```python
from build123d import *

# Parameters (mm, degrees)
SKETCH1_W           = 25.4
SKETCH1_H           = 88.9
BOSS_EXTRUDE1_DEPTH = 30.226
SKETCH2_R           = 3.175
CUT_EXTRUDE1_DEPTH  = 12.7
SKETCH3_R           = 8.763
CUT_EXTRUDE2_DEPTH  = 3.556
CUT_EXTRUDE3_START  = -21.844
SKETCH4_R           = 10.795
CUT_EXTRUDE3_DEPTH  = 21.844
SKETCH5_W           = 54.61
SKETCH5_H           = 30.226
BOSS_EXTRUDE2_DEPTH = 3.175
SKETCH6_R           = 1.5875
CUT_EXTRUDE4_DEPTH  = 3.175
BOSS_EXTRUDE3_START = 2.54
SKETCH8_R           = 10.795
SKETCH8_R_2         = 6.35
BOSS_EXTRUDE3_DEPTH = 2.54


with BuildPart() as part:
    # Sketch1 → Boss-Extrude1 (new body)
    with BuildSketch(Plane.XY):
        Rectangle(SKETCH1_W, SKETCH1_H)
    extrude(amount=BOSS_EXTRUDE1_DEPTH)

    # Sketch2 → Cut-Extrude1 (cut)
    with BuildSketch(Plane(origin=(12.7, 0, 0), x_dir=(0, 0, -1), z_dir=(1, 0, 0))):
        with Locations((-15.113, 38.1)):
            Circle(SKETCH2_R)
        with Locations((-15.113, -38.1)):
            Circle(SKETCH2_R)
    extrude(amount=-CUT_EXTRUDE1_DEPTH, mode=Mode.SUBTRACT)

    # Sketch3 → Cut-Extrude2 (cut)
    with BuildSketch(Plane(origin=(12.7, 0, 0), x_dir=(0, 0, -1), z_dir=(1, 0, 0))):
        with Locations((-15.113, 0)):
            Circle(SKETCH3_R)
    extrude(amount=-CUT_EXTRUDE2_DEPTH, mode=Mode.SUBTRACT)

    # Sketch4 → Cut-Extrude3 (cut)
    with BuildSketch(Plane(origin=(9.144, 0, 0), x_dir=(0, 0, -1), z_dir=(1, 0, 0)).offset(CUT_EXTRUDE3_START)):
        with Locations((-15.113, 0)):
            Circle(SKETCH4_R)
    extrude(amount=CUT_EXTRUDE3_DEPTH, mode=Mode.SUBTRACT)

    # Sketch5 → Boss-Extrude2 (add)
    with BuildSketch(Plane.XZ.offset(44.45)):
        with Locations((0, 15.113)):
            Rectangle(SKETCH5_W, SKETCH5_H)
    extrude(amount=BOSS_EXTRUDE2_DEPTH)

    # Sketch6 → Cut-Extrude4 (cut)
    with BuildSketch(Plane.XZ.offset(47.625)):
        with Locations(Location((-23.495, 25.908, 0), (0, 0, 270))):
            Circle(SKETCH6_R)
        with Locations(Location((-23.495, 4.318, 0), (0, 0, 270))):
            Circle(SKETCH6_R)
        with Locations(Location((23.495, 4.318, 0), (0, 0, 270))):
            Circle(SKETCH6_R)
        with Locations(Location((23.495, 25.908, 0), (0, 0, 270))):
            Circle(SKETCH6_R)
    extrude(amount=-CUT_EXTRUDE4_DEPTH, mode=Mode.SUBTRACT)

    # Sketch8 → Boss-Extrude3 (add)
    with BuildSketch(Plane.ZY.offset(-9.144).offset(BOSS_EXTRUDE3_START)):
        with Locations(Location((15.113, 0, 0), (0, 0, 180))):
            Circle(SKETCH8_R)
        with Locations((15.113, 0)):
            Circle(SKETCH8_R_2, mode=Mode.SUBTRACT)
    extrude(amount=-BOSS_EXTRUDE3_DEPTH)


solid = part.part
```
For this review, take the finished solid that the model builds, in its own axes (mm). A direction names the side the tool comes from. Round coordinates to 2 decimals unless told otherwise and drop trailing zeros. Loops run counter-clockwise (first coordinate to the right, second up) from the corner with the lowest first, then second, coordinate; pieces in that order, holes last.
(1) We need section C-C (y = -38.1). Give the boundary of the cut face in (x, z).
Returned:
outline: (-12.7, 0) - (12.7, 0) - (12.7, 11.94) - (0, 11.94) - (0, 18.29) - (12.7, 18.29) - (12.7, 30.23) - (-12.7, 30.23) - close
(2) Tool access review of faces 4 (the flat face through (12.7, -11, 15)), 5 (the cylindrical face through (6.439, 38.24, 18.285)), 6 (the flat face through (-12.7, -11, 18)): name each direction out of +Z, -Z, +X, -X, +Y, -Y from which nothing blocks a thin tool from reaching the whole face with its end or side.
Returned:
face 4: +Z, -Z, +X, +Y
face 5: +X
face 6: +Z, -Z, -X, +Y
(3) Wall thickness on line 1 along Z through (x, y) = (-5, 0); line 2 along Y through (x, z) = (-13, 15) (3 decimals); line 3 along Y through (x, z) = (-3, 19) (3 decimals): over which ranges is each line inside the solid? List them lowest first.
Returned:
line 1: z = 0 to 4.32, 25.91 to 30.23
line 2: y = -47.625 to -44.45
line 3: y = -47.625 to -10.071, 10.071 to 44.45
(4) We need section D-D (x = -18.5). Give the boundary of the cut face in (y, z) (3 decimals).
Returned:
outline: (-47.625, 0) - (-44.45, 0) - (-44.45, 30.226) - (-47.625, 30.226) - close
(5) Clearance check with flat-ended pins moving along their axes: P1, Ø17.5, axis at y = 4.5, z = 19.5, coming from the -X side; P2, Ø4, axis at x = 23.495, z = 4.318, coming from the +Y side; P3, Ø9, axis at y = -4, z = 18.5, coming from the +X side; P4, Ø2.5, axis at x = -23.495, z = 25.908, coming from the +Y side. State where each tip first meets the part, or that it passes through.
Returned:
P1: stops at x = -12.7
P2: stops at y = -44.45
P3: stops at x = 12.7
P4: passes through
(6) We need section A-A (y = 0). Give the boundary of the cut face in (x, z).
Returned:
outline: (-12.7, 0) - (12.7, 0) - (12.7, 6.35) - (9.14, 6.35) - (9.14, 8.76) - (6.6, 8.76) - (6.6, 4.32) - (-12.7, 4.32) - close; (-12.7, 25.91) - (6.6, 25.91) - (6.6, 21.46) - (9.14, 21.46) - (9.14, 23.88) - (12.7, 23.88) - (12.7, 30.23) - (-12.7, 30.23) - close
(7) Mouldability with a two-part tool opening along X and no side actions: class faces 1 (the flat face through (0, 38, 15)), 2 (the cylindrical face through (24.83, -46.06, 25.05)), 3 (the flat face through (6.604, 5, 10)) as released by +X, released by -X, zero draft, split by the parting line, or undercut.
Returned:
face 1: released by +X
face 2: undercut
face 3: released by -X
(8) We need section B-B (x = 11). Give the boundary of the cut face in (y, z) (3 decimals), plus the area to 3 significant figures.
Returned:
outline: (-47.625, 0) - (44.45, 0) - (44.45, 30.226) - (-47.625, 30.226) - close; hole circle Ø6.35 at (-38.1, 15.113); hole circle Ø17.526 at (0, 15.113); hole circle Ø6.35 at (38.1, 15.113)
area: 2,480 mm2
